```python
from build123d import *

# Parameters (mm, degrees)
SKETCH_2_R          = 2.6
SKETCH_2_R_2        = 1.75
EXTRUDE_3_DEPTH     = 2
EXTRUDE_START       = -2
SKETCH_3_R          = 2.6
EXTRUDE_4_DEPTH     = 2
EXTRUDE_5_DEPTH     = 2
FILLET_1_R          = 6
CUT_EXTRUDE_1_DEPTH = 2
EXTRUDE_6_DEPTH     = 2
SKETCH_8_W          = 26
SKETCH_8_H          = 9
EXTRUDE_7_DEPTH     = 2


with BuildPart() as part:
    # 草图2 → 凸台-拉伸3 (new body)
    with BuildSketch(Plane(origin=(0, 0, 0), x_dir=(1, 0, 0), z_dir=(0, 1, 0))):
        Polygon((15, 14), (-1.25, 14), (-1.25, 31.003525978), (-10.75, 31.003525978), (-10.75, 19.003525978), (-37.293472201, 19.003525978), (-37.293472201, 10.003525978), (-23.25, 10.003525978), (-23.25, -3.996474022), (-13.75, -3.996474022), (15, -3.996474022), (17.373946176, -3.996474022), (17.373946176, 14), align=None)
        with Locations(Location((-18.5, 1.003525978, 0), (0, 0, 270))):
            Circle(SKETCH_2_R, mode=Mode.SUBTRACT)
        with Locations(Location((0, 0.053173587, 0), (0, 0, 270))):
            Circle(SKETCH_2_R_2, mode=Mode.SUBTRACT)
        with Locations(Location((15, 0.053173587, 0), (0, 0, 270))):
            Circle(SKETCH_2_R_2, mode=Mode.SUBTRACT)
        with Locations(Location((0, 10.053173587, 0), (0, 0, 270))):
            Circle(SKETCH_2_R_2, mode=Mode.SUBTRACT)
        with Locations(Location((15, 10.053173587, 0), (0, 0, 270))):
            Circle(SKETCH_2_R_2, mode=Mode.SUBTRACT)
        with Locations(Location((-6, 26.003525978, 0), (0, 0, 270))):
            Circle(SKETCH_2_R, mode=Mode.SUBTRACT)
    extrude(amount=EXTRUDE_3_DEPTH)

    # 草图3 → 凸台-拉伸4 (add)
    # profile 1 of 9: a face of its own
    with BuildSketch(Plane(origin=(0, 2, 0), x_dir=(1, 0, 0), z_dir=(0, 1, 0)).offset(EXTRUDE_START)):
        with BuildLine():
            Line((-1.25, 31.003525978), (-10.75, 31.003525978))
            Line((-10.75, 31.003525978), (-10.75, 21.003525978))
            ThreePointArc((-10.75, 21.003525978), (-8.557314455, 19.59863388), (-6, 19.106968866))
            ThreePointArc((-6, 19.106968866), (-3.442685545, 19.59863388), (-1.25, 21.003525978))
            Line((-1.25, 21.003525978), (-1.25, 31.003525978))
        make_face()
        with Locations(Location((-6, 26.003525978, 0), (0, 0, 270))):
            Circle(SKETCH_3_R, mode=Mode.SUBTRACT)
    # profile 2 of 9: a face of its own
    with BuildSketch(Plane(origin=(0, 2, 0), x_dir=(1, 0, 0), z_dir=(0, 1, 0)).offset(EXTRUDE_START)):
        with BuildLine():
            ThreePointArc((-10.75, 21.003525978), (-12.895048442, 25.85927974), (-10.9549552, 30.800495747))
            Line((-10.9549552, 30.800495747), (-14.196613842, 27.452074948))
            ThreePointArc((-14.196613842, 27.452074948), (-23.307699904, 21.20281017), (-34.134904, 19.003525978))
            Line((-34.134904, 19.003525978), (-10.75, 19.003525978))
            Line((-10.75, 19.003525978), (-10.75, 21.003525978))
        make_face()
    # profile 3 of 9: a face of its own
    with BuildSketch(Plane(origin=(0, 2, 0), x_dir=(1, 0, 0), z_dir=(0, 1, 0)).offset(EXTRUDE_START)):
        with BuildLine():
            ThreePointArc((-1.25, 31.003525978), (-6, 32.90008309), (-10.75, 31.003525978))
            Line((-10.75, 31.003525978), (-1.25, 31.003525978))
        make_face()
    # profile 4 of 9: a face of its own
    with BuildSketch(Plane(origin=(0, 2, 0), x_dir=(1, 0, 0), z_dir=(0, 1, 0)).offset(EXTRUDE_START)):
        with BuildLine():
            ThreePointArc((0.896557112, 26.003525978), (0.337237027, 28.72417422), (-1.25, 31.003525978))
            Line((-1.25, 31.003525978), (-1.25, 21.003525978))
            ThreePointArc((-1.25, 21.003525978), (0.337237027, 23.282877735), (0.896557112, 26.003525978))
        make_face()
    # profile 5 of 9: a face of its own
    with BuildSketch(Plane(origin=(0, 2, 0), x_dir=(1, 0, 0), z_dir=(0, 1, 0)).offset(EXTRUDE_START)):
        with BuildLine():
            Line((-26.624271801, 4.358914994), (-25.133517426, -0.882991066))
            ThreePointArc((-25.133517426, -0.882991066), (-25.152228686, 2.822963667), (-23.25, 6.003525978))
            Line((-23.25, 6.003525978), (-23.25, 10.003525978))
            Line((-23.25, 10.003525978), (-34.097989538, 10.003525978))
            ThreePointArc((-34.097989538, 10.003525978), (-29.415092732, 8.433817083), (-26.624271801, 4.358914994))
        make_face()
    # profile 6 of 9: a face of its own
    with BuildSketch(Plane(origin=(0, 2, 0), x_dir=(1, 0, 0), z_dir=(0, 1, 0)).offset(EXTRUDE_START)):
        with BuildLine():
            ThreePointArc((-11.603442888, 1.003525978), (-15.779351758, 7.340763005), (-23.25, 6.003525978))
            Line((-23.25, 6.003525978), (-23.25, -3.996474022))
            Line((-23.25, -3.996474022), (-13.75, -3.996474022))
            ThreePointArc((-13.75, -3.996474022), (-12.162762973, -1.717122265), (-11.603442888, 1.003525978))
        make_face()
        with Locations(Location((-18.5, 1.003525978, 0), (0, 0, 270))):
            Circle(SKETCH_3_R, mode=Mode.SUBTRACT)
    # profile 7 of 9: a face of its own
    with BuildSketch(Plane(origin=(0, 2, 0), x_dir=(1, 0, 0), z_dir=(0, 1, 0)).offset(EXTRUDE_START)):
        with BuildLine():
            ThreePointArc((-23.25, 6.003525978), (-25.152228686, 2.822963667), (-25.133517426, -0.882991066))
            ThreePointArc((-25.133517426, -0.882991066), (-24.400810222, -2.566199323), (-23.25, -3.996474022))
            Line((-23.25, -3.996474022), (-23.25, 6.003525978))
        make_face()
    # profile 8 of 9: a face of its own
    with BuildSketch(Plane(origin=(0, 2, 0), x_dir=(1, 0, 0), z_dir=(0, 1, 0)).offset(EXTRUDE_START)):
        with BuildLine():
            Line((-13.75, -3.996474022), (-23.25, -3.996474022))
            ThreePointArc((-23.25, -3.996474022), (-18.5, -5.893031134), (-13.75, -3.996474022))
        make_face()
    # profile 9 of 9: a face of its own
    with BuildSketch(Plane(origin=(0, 2, 0), x_dir=(1, 0, 0), z_dir=(0, 1, 0)).offset(EXTRUDE_START)):
        with BuildLine():
            ThreePointArc((-10.75, 31.003525978), (-10.853539345, 30.903082674), (-10.9549552, 30.800495747))
            ThreePointArc((-10.9549552, 30.800495747), (-12.895048442, 25.85927974), (-10.75, 21.003525978))
            Line((-10.75, 21.003525978), (-10.75, 31.003525978))
        make_face()
    extrude(amount=EXTRUDE_4_DEPTH)

    # 草图4 → 凸台-拉伸5 (add)
    with BuildSketch(Plane.XZ):
        with BuildLine():
            ThreePointArc((-1.25, -21.003525978), (0.561593491, -23.880323006), (0.778699813, -27.273064812))
            Line((0.778699813, -27.273064812), (3.023667629, -17.033583157))
            ThreePointArc((3.023667629, -17.033583157), (4.374639496, -14.852535674), (6.79440726, -14))
            Line((6.79440726, -14), (-1.25, -14))
            Line((-1.25, -14), (-1.25, -21.003525978))
        make_face()
    extrude(amount=-EXTRUDE_5_DEPTH)

    # 圆角1
    fillet_1_edges = [part.edges().sort_by_distance(p)[0] for p in [
        (-13.75, 1, 3.996474022),
    ]]
    fillet(fillet_1_edges, radius=FILLET_1_R)

    # 草图6 → 切除-拉伸1 (cut)
    with BuildSketch(Plane(origin=(0, 2, 0), x_dir=(1, 0, 0), z_dir=(0, 1, 0))):
        with BuildLine():
            Line((-32.293472201, 12.903525978), (-9.293472201, 12.903525978))
            ThreePointArc((-9.293472201, 12.903525978), (-7.693472201, 14.503525978), (-9.293472201, 16.103525978))
            Line((-9.293472201, 16.103525978), (-32.293472201, 16.103525978))
            ThreePointArc((-32.293472201, 16.103525978), (-33.893472201, 14.503525978), (-32.293472201, 12.903525978))
        make_face()
    extrude(amount=-CUT_EXTRUDE_1_DEPTH, mode=Mode.SUBTRACT)

    # 草图7 → 凸台-拉伸6 (add)
    with BuildSketch(Plane(origin=(0, 2, 0), x_dir=(1, 0, 0), z_dir=(0, 1, 0))):
        with BuildLine():
            Line((19.085277426, 12.28866875), (19.085277426, -2.285142773))
            ThreePointArc((19.085277426, -2.285142773), (18.584040107, -3.495236704), (17.373946176, -3.996474022))
            Line((17.373946176, -3.996474022), (17.373946176, 14))
            ThreePointArc((17.373946176, 14), (18.584040107, 13.498762682), (19.085277426, 12.28866875))
        make_face()
    extrude(amount=-EXTRUDE_6_DEPTH)

    # 草图8 → 凸台-拉伸7 (add)
    with BuildSketch(Plane(origin=(0, 2, 0), x_dir=(1, 0, 0), z_dir=(0, 1, 0))):
        with Locations((-50.293472201, 14.503525978)):
            Rectangle(SKETCH_8_W, SKETCH_8_H)
        with BuildLine():
            ThreePointArc((-39.293472201, 12.903525978), (-37.693472201, 14.503525978), (-39.293472201, 16.103525978))
            Line((-39.293472201, 16.103525978), (-59.293472201, 16.103525978))
            ThreePointArc((-59.293472201, 16.103525978), (-60.893472201, 14.503525978), (-59.293472201, 12.903525978))
            Line((-59.293472201, 12.903525978), (-39.293472201, 12.903525978))
        make_face(mode=Mode.SUBTRACT)
    extrude(amount=-EXTRUDE_7_DEPTH)


solid = part.part
```
Could you check a few things on this model? Use its own coordinates, in mm. A direction names the side the tool comes from. Round coordinates to 2 decimals unless told otherwise and drop trailing zeros. Order: outer loops, then holes, each group sorted by start corner. A loop starts at its lowest first (then second) coordinate and runs counter-clockwise, first axis right, second up. Notation, with made-up numbers: M 40.25,82.25 L 83.25,82.25 A11 cw 83.25,100.25 Z; hole C -30.75,68.5 d10. An arc over 180 degrees is marked long. One line per question, with ' | ' between items. Start each with the question number.
(1) Please list where these lines run through material, in increasing order: line 1 along X through (y, z) = (0.7, 0.5); line 2 along Z through (x, y) = (-58.5, 1.65); line 3 along X through (y, z) = (0.5, -15.5).
(2) Thinking about a two-plate mould opening in Z: for faces 5 (the face through (-12.6, 1, -29.1)), 6 (the face through (-29.471, 0.986, -8.476)), 7 (the face through (-37.694, 1.014, -14.468)), which applies, +Z half, -Z half, draft (parallel to the pull), parting line (faces both ways), or undercut?
(3) Suppose I cut it at D-D on x = -52.5. List the corners of the cut face in (y, z) for me.
(4) For P1, Ø0.6, axis at x = 10.5, y = 1.5, coming from the -Z side; P2, Ø0.6, axis at x = -54, y = 1, coming from the -Z side; P3, Ø1, axis at x = -48, y = 1, coming from the +Z side, each with a flat end and sliding along its axis, tell me the tip position at first contact or that it passes through.
(5) For faces 1 (the face through (3, 1, 3.996)), 2 (the face through (12, 1, -14)), 3 (the face through (-14, 2, -9)), 4 (the face through (-33.893, 1.014, -14.539)), which set-ups out of +Z, -Z, +X, -X, +Y, -Y let a thin tool reach every point of the face, with its end or its side?
(6) Suppose I cut it at B-B on x = 15. List the corners of the cut face in (y, z) for me, then the cut area to 3 significant figures.
(7) Suppose I cut it at A-A on x = -6. List the corners of the cut face in (y, z) for me, then the cut area to 3 significant figures.
(8) Suppose I cut it at C-C on y = 0.3. Count the separate pieces of the cut face and the enclosed holes in it, then the cut area to 3 significant figures.
Geometry results:
1) line 1: -25.24 to -20.62, -16.38 to -1.66, 1.66 to 13.34, 16.66 to 19.09 | line 2: -19 to -16.1, -12.9 to -10 | line 3: -63.29 to -60.55, -38.04 to -33.55, -8.04 to 3.74
2) face 5: -Z half | face 6: +Z half | face 7: undercut
3) outline: M 0,-19 L 2,-19 L 2,-16.1 L 0,-16.1 Z; M 0,-12.9 L 2,-12.9 L 2,-10 L 0,-10 Z
4) P1: z = -14 | P2: z = -19 | P3: z = -10
5) face 1: +Z, +X, +Y, -Y | face 2: -Z, +X, +Y, -Y | face 3: +Z, -Z, +X, -X, +Y | face 4: +Y, -Y
6) outline: M 0,-14 L 2,-14 L 2,-11.8 L 0,-11.8 Z; M 0,-8.3 L 2,-8.3 L 2,-1.8 L 0,-1.8 Z; M 0,1.7 L 2,1.7 L 2,4 L 0,4 Z | area: 22.0 mm²
7) outline: M 0,-32.9 L 2,-32.9 L 2,-28.6 L 0,-28.6 Z; M 0,-23.4 L 2,-23.4 L 2,4 L 0,4 Z | area: 63.4 mm²
8) separate pieces: 1 | enclosed holes: 8 | area: 1,320 mm²
